from build123d import *

# Parameters (mm, degrees)
F0_R     = 20.37
F0_R_2   = 6.4
F0_R_3   = 2.55
F1_DEPTH = 1.2
F2_DEPTH = 5.7
F3_R     = 0.3


# Not quite as in the source:
# - a feature names something its author has since deleted; it is built from what else it names


with BuildPart() as f1:
    # F0 (on Top) → F1 (new body)
    with BuildSketch(Plane.XY):
        Circle(F0_R)
        Circle(F0_R_2, mode=Mode.SUBTRACT)
        Circle(F0_R_2)
        Circle(F0_R_3, mode=Mode.SUBTRACT)
    extrude(amount=-F1_DEPTH)

    # F0 (on Top) → F2 (join)
    with BuildSketch(Plane.XY):
        Circle(F0_R_2)
        Circle(F0_R_3, mode=Mode.SUBTRACT)
    extrude(amount=F2_DEPTH)

    # F3
    f3_edges = [f1.edges().sort_by_distance(p)[0] for p in [
        (-20.37, 0, -1.2),
        (-6.4, 0, 5.7),
    ]]
    fillet(f3_edges, radius=F3_R)


solid = f1.part
Source: CAD feature listing. Evaluate the final solid. Frame: model axes, mm. A direction names the side the tool comes from. Give positions to 0.01 mm unless a question says otherwise; leave off trailing zeros. Loops run counter-clockwise (first coordinate to the right, second up) from the corner with the lowest first, then second, coordinate; pieces in that order, holes last. Notation, with made-up numbers: (33.5, 78.25) -> (73.5, 78.25) arc R17 cw to (73.5, 108.25) -> close; hole circle Ø3 at (83.25, 21.5). An arc over 180 degrees is marked (long way). Use a Markdown table: item, result. Add a question column.
1) Reachability of faces 1 (the face through (-5.08, -3.89, 2.66)), 2 (the face through (10.951, 17.176, -0.444)) from +Z, -Z, +X, -X, +Y, -Y: full face, straight path, thin tool, end or side. Return the list, or none.
2) Line query: line 1 along Y through (x, z) = (0, 1.75); line 2 along Z through (x, y) = (12.5, 9); line 3 along Y through (x, z) = (1.5, 1.75). Output: solid intervals per line, ascending. Write a range as [from, to].
3) Section query A-A, the plane x = 0. Return the cut outline in (y, z), then the cut area to 3 significant figures.
4) First-contact query: pin 1 (4 mm diameter, centred on x = -3, z = 1, fed in from +Y); pin 2 (6 mm diameter, centred on x = 0, y = 0, fed in from +Z); pin 3 (4 mm diameter, centred on x = 4.5, z = 4.5, fed in from -Y); pin 4 (2 mm diameter, centred on x = 13, z = 0, fed in from -Y). Flat tips, straight axial feed; report the tip coordinate or a pass-through.
5) Section query C-C, the plane z = 0.75. Return the cut outline in (x, y), then the cut area to 3 significant figures.
Numbers:
| question | item | result |
|---|---|---|
| 1 | face 1 | +Z |
| 1 | face 2 | +Z, -Z |
| 2 | line 1 | y = [-6.4, -2.55], [2.55, 6.4] |
| 2 | line 2 | z = [-1.2, 0] |
| 2 | line 3 | y = [-6.22, -2.06], [2.06, 6.22] |
| 3 | outline | (-20.37, -0.9) arc R0.3 ccw to (-20.07, -1.2) -> (-2.55, -1.2) -> (-2.55, 5.7) -> (-6.1, 5.7) arc R0.3 ccw to (-6.4, 5.4) -> (-6.4, 0) -> (-20.37, 0) -> close; (2.55, -1.2) -> (20.07, -1.2) arc R0.3 ccw to (20.37, -0.9) -> (20.37, 0) -> (6.4, 0) -> (6.4, 5.4) arc R0.3 ccw to (6.1, 5.7) -> (2.55, 5.7) -> close |
| 3 | area | 86.6 mm2 |
| 4 | pin 1 | stops at y = 20.33 |
| 4 | pin 2 | stops at z = 5.7 |
| 4 | pin 3 | stops at y = -5.89 |
| 4 | pin 4 | stops at y = -16.46 |
| 5 | outline | circle Ø12.8 at (0, 0); hole circle Ø5.1 at (0, 0) |
| 5 | area | 108 mm2 |
